Source: CAD feature listing. Evaluate the final solid. Frame: model axes, mm. Face numbers are marked on the shaded views. Give positions to 0.01 mm unless a question says otherwise; leave off trailing zeros. Loops run counter-clockwise (first coordinate to the right, second up) from the corner with the lowest first, then second, coordinate; pieces in that order, holes last. Notation, with made-up numbers: (32.5, 63.5) - (40.5, 63.5) arc R32 cw to (40.5, 98.5) - close; hole circle Ø11 at (-40, 58). An arc over 180 degrees is marked (long way). Put each result on its own line as item: value.
```python
from build123d import *

# Parameters (mm, degrees)
F1_DEPTH = 8
F2_DEPTH = 2
F3_W     = 30
F3_H     = 3
F4_DEPTH = 10
F5_R     = 1
F6_SIZE  = 1


with BuildPart() as f1:
    # F0 (on Top) → F1 (new body)
    with BuildSketch(Plane.XY):
        with BuildLine():
            Line((-57.5, -64.5), (57.5, -64.5))
            ThreePointArc((57.5, -64.5), (62.449747, -62.449747), (64.5, -57.5))
            Line((64.5, -57.5), (64.5, 57.5))
            ThreePointArc((64.5, 57.5), (62.449747, 62.449747), (57.5, 64.5))
            Line((57.5, 64.5), (-57.5, 64.5))
            ThreePointArc((-57.5, 64.5), (-62.449747, 62.449747), (-64.5, 57.5))
            Line((-64.5, 57.5), (-64.5, -57.5))
            ThreePointArc((-64.5, -57.5), (-62.449747, -62.449747), (-57.5, -64.5))
        make_face()
        with BuildLine():
            ThreePointArc((-57.5, -62.7), (-61.176955, -61.176955), (-62.7, -57.5))
            Line((-62.7, -57.5), (-62.7, 57.5))
            ThreePointArc((-62.7, 57.5), (-61.176955, 61.176955), (-57.5, 62.7))
            Line((-57.5, 62.7), (57.5, 62.7))
            ThreePointArc((57.5, 62.7), (61.176955, 61.176955), (62.7, 57.5))
            Line((62.7, 57.5), (62.7, -57.5))
            ThreePointArc((62.7, -57.5), (61.176955, -61.176955), (57.5, -62.7))
            Line((57.5, -62.7), (-57.5, -62.7))
        make_face(mode=Mode.SUBTRACT)
    extrude(amount=F1_DEPTH)

    # F0 (on Top) → F2 (join)
    with BuildSketch(Plane.XY):
        with BuildLine():
            Line((-62.7, 57.5), (-62.7, -57.5))
            ThreePointArc((-62.7, -57.5), (-61.176955, -61.176955), (-57.5, -62.7))
            Line((-57.5, -62.7), (57.5, -62.7))
            ThreePointArc((57.5, -62.7), (61.176955, -61.176955), (62.7, -57.5))
            Line((62.7, -57.5), (62.7, 57.5))
            ThreePointArc((62.7, 57.5), (61.176955, 61.176955), (57.5, 62.7))
            Line((57.5, 62.7), (-57.5, 62.7))
            ThreePointArc((-57.5, 62.7), (-61.176955, 61.176955), (-62.7, 57.5))
        make_face()
    extrude(amount=F2_DEPTH)

    # F3 (on face) → F4 (join)
    with BuildSketch(Plane.XZ.offset(64.5)):
        with Locations((0, 1.5)):
            Rectangle(F3_W, F3_H)
    extrude(amount=F4_DEPTH)

    # F5
    f5_edges = [f1.edges().sort_by_distance(p)[0] for p in [
        (0, -74.5, 0),
        (0, -74.5, 3),
    ]]
    fillet(f5_edges, radius=F5_R)

    # F6
    f6_edges = [f1.edges().sort_by_distance(p)[0] for p in [
        (0, 62.7, 8),
        (-61.176955, 61.176955, 8),
        (-62.7, 0, 8),
        (-61.176955, -61.176955, 8),
        (0, -62.7, 8),
        (61.176955, -61.176955, 8),
        (62.7, 0, 8),
        (61.176955, 61.176955, 8),
    ]]
    chamfer(f6_edges, length=F6_SIZE)


solid = f1.part
```
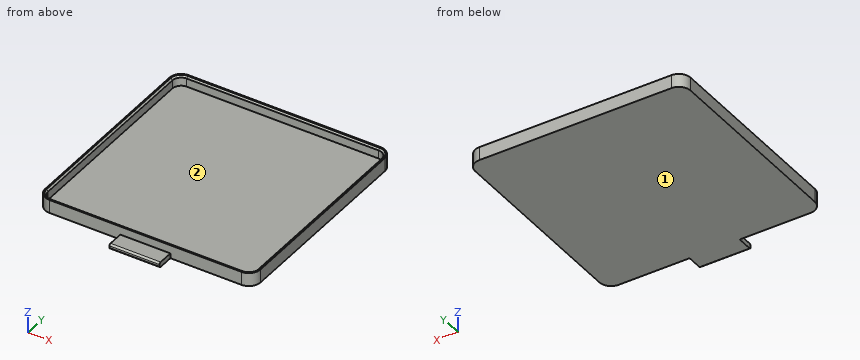
1) Section query A-A, the plane z = 4.25. Output: boundary loops of the cut face in (x, y).
Check result:
outline: (-64.5, -57.5) arc R7 ccw to (-57.5, -64.5) - (57.5, -64.5) arc R7 ccw to (64.5, -57.5) - (64.5, 57.5) arc R7 ccw to (57.5, 64.5) - (-57.5, 64.5) arc R7 ccw to (-64.5, 57.5) - close; hole (-62.7, -57.5) arc R5.2 ccw to (-57.5, -62.7) - (57.5, -62.7) arc R5.2 ccw to (62.7, -57.5) - (62.7, 57.5) arc R5.2 ccw to (57.5, 62.7) - (-57.5, 62.7) arc R5.2 ccw to (-62.7, 57.5) - close
2) Pin query (flat end, axial travel): P1, Ø1.5, axis at x = -44.5, z = 4.5, coming from the -Y side; P2, Ø3.5, axis at y = -67.5, z = 1.5, coming from the -X side; P3, Ø7, axis at x = -6.5, y = -70, coming from the +Z side. Return the tip coordinate at first contact, or that it passes through.
Check result:
P1: y = -64.5
P2: x = -15
P3: z = 3
3) Section query C-C, the plane x = 9. Output: boundary loops of the cut face in (y, z).
Check result:
outline: (-74.5, 1) arc R1 ccw to (-73.5, 0) - (64.5, 0) - (64.5, 8) - (63.7, 8) - (62.7, 7) - (62.7, 2) - (-62.7, 2) - (-62.7, 7) - (-63.7, 8) - (-64.5, 8) - (-64.5, 3) - (-73.5, 3) arc R1 ccw to (-74.5, 2) - close
4) Section query B-B, the plane y = -23.5. Output: boundary loops of the cut face in (x, z), plus the area to 3 significant figures.
Check result:
outline: (-64.5, 0) - (64.5, 0) - (64.5, 8) - (63.7, 8) - (62.7, 7) - (62.7, 2) - (-62.7, 2) - (-62.7, 7) - (-63.7, 8) - (-64.5, 8) - close
area: 279 mm²
5) Material intervals for line 1 along Y through (x, z) = (36, 2.5); line 2 along Y through (x, z) = (41.5, 1), sorted ascending. Write a range as [from, to].
Check result:
line 1: [-64.5, -62.7], [62.7, 64.5]
line 2: [-64.5, 64.5]
6) Mould query, pull axis Y, two halves, no side actions, for the marked faces 1 and 2. Classes: pulls with the +Y half, pulls with the -Y half, needs draft (parallel to the pull), parting line crosses it, or undercut.
Check result:
face 1: needs draft
face 2: undercut
